Check sheet for the modelled part. Datum: model origin and axes. Units: mm. A direction names the side the tool comes from. Round coordinates to 2 decimals unless told otherwise and drop trailing zeros. Order: outer loops, then holes, each group sorted by start corner. A loop starts at its lowest first (then second) coordinate and runs counter-clockwise, first axis right, second up. Notation, with made-up numbers: (68.5, -28) -> (117.5, -28) arc R17 ccw to (117.5, -20) -> close; hole circle Ø1 at (-39.75, 12). An arc over 180 degrees is marked (long way). Answer in a Markdown table with one row per item.
```python
from build123d import *

# Parameters (mm, degrees)
SKETCH1_R           = 3.75
BOSS_EXTRUDE1_DEPTH = 8
SKETCH3_R           = 3.75
SKETCH3_R_2         = 3.25
CUT_EXTRUDE1_DEPTH  = 2
SKETCH4_R           = 1.75
CUT_EXTRUDE2_DEPTH  = 7.5
SKETCH5_R           = 2.5
CUT_EXTRUDE3_DEPTH  = 1


with BuildPart() as part:
    # Sketch1 → Boss-Extrude1 (new body)
    with BuildSketch(Plane(origin=(0, 0, 0), x_dir=(1, 0, 0), z_dir=(0, 1, 0))):
        Circle(SKETCH1_R)
    extrude(amount=BOSS_EXTRUDE1_DEPTH)

    # Sketch3 → Cut-Extrude1 (cut)
    with BuildSketch(Plane(origin=(0, 8, 0), x_dir=(1, 0, 0), z_dir=(0, 1, 0))):
        Circle(SKETCH3_R)
        Circle(SKETCH3_R_2, mode=Mode.SUBTRACT)
    extrude(amount=-CUT_EXTRUDE1_DEPTH, mode=Mode.SUBTRACT)

    # Sketch4 → Cut-Extrude2 (cut)
    with BuildSketch(Plane(origin=(0, 8, 0), x_dir=(1, 0, 0), z_dir=(0, 1, 0))):
        Circle(SKETCH4_R)
    extrude(amount=-CUT_EXTRUDE2_DEPTH, mode=Mode.SUBTRACT)

    # Sketch5 → Cut-Extrude3 (cut)
    with BuildSketch(Plane(origin=(0, 8, 0), x_dir=(1, 0, 0), z_dir=(0, 1, 0))):
        Circle(SKETCH5_R)
    extrude(amount=-CUT_EXTRUDE3_DEPTH, mode=Mode.SUBTRACT)


solid = part.part
```
(1) Section check B-B on y = 2. Record the boundary of the cut face in (x, z), plus the area to 3 significant figures.
Solutions:
| item | result |
|---|---|
| outline | circle Ø7.5 at (0, 0); hole circle Ø3.5 at (0, 0) |
| area | 34.6 mm^2 |
(2) Section check D-D on z = 2.75. Record the boundary of the cut face in (x, y).
Solutions:
| item | result |
|---|---|
| outline | (-2.55, 0) -> (2.55, 0) -> (2.55, 6) -> (1.73, 6) -> (1.73, 8) -> (-1.73, 8) -> (-1.73, 6) -> (-2.55, 6) -> close |
(3) Section check A-A on x = 0. Record the boundary of the cut face in (y, z).
Solutions:
| item | result |
|---|---|
| outline | (0, -3.75) -> (6, -3.75) -> (6, -3.25) -> (8, -3.25) -> (8, -2.5) -> (7, -2.5) -> (7, -1.75) -> (0.5, -1.75) -> (0.5, 1.75) -> (7, 1.75) -> (7, 2.5) -> (8, 2.5) -> (8, 3.25) -> (6, 3.25) -> (6, 3.75) -> (0, 3.75) -> close |
(4) Scan lines: probe 1 along Z at (x, y) = (0, 7.7); probe 2 along X at (y, z) = (1.25, 0). Record each from-to range of solid material in increasing order. Write a range as from..to.
Solutions:
| item | result |
|---|---|
| probe 1 | -3.25..-2.5, 2.5..3.25 |
| probe 2 | -3.75..-1.75, 1.75..3.75 |
(5) Draft check along Z on faces 1 (the flat face through (-1.4, 6, -3.1)), 2 (the cylindrical face through (-2.579, 7.014, 1.978)), 3 (the cylindrical face through (1.617, 3.796, 0.67)). Enter one of: pulls with the +Z half, pulls with the -Z half, needs draft (parallel to the pull), parting line crosses it, or undercut.
Solutions:
| item | result |
|---|---|
| face 1 | needs draft |
| face 2 | parting line crosses it |
| face 3 | undercut |
(6) Section check C-C on z = 0. Record the boundary of the cut face in (x, y), plus the area to 4 significant figures.
Solutions:
| item | result |
|---|---|
| outline | (-3.75, 0) -> (3.75, 0) -> (3.75, 6) -> (3.25, 6) -> (3.25, 8) -> (2.5, 8) -> (2.5, 7) -> (1.75, 7) -> (1.75, 0.5) -> (-1.75, 0.5) -> (-1.75, 7) -> (-2.5, 7) -> (-2.5, 8) -> (-3.25, 8) -> (-3.25, 6) -> (-3.75, 6) -> close |
| area | 30.25 mm^2 |
(7) Tool access check on faces 4 (the cylindrical face through (-0.54, 7.51, 2.44)), 5 (the flat face through (2, 8, 2)). Record the directions out of +Z, -Z, +X, -X, +Y, -Y that give a thin tool (end or side, any length) a straight path to the whole face; none if there is none.
Solutions:
| item | result |
|---|---|
| face 4 | +Y |
| face 5 | +Z, -Z, +X, -X, +Y |
(8) Depth check by flat-ended pin: pin 1 Ø3 at (x, y) = (3, 5) entering from -Z; pin 2 Ø4 at (x, y) = (2.5, 4.5) entering from -Z; pin 3 Ø4 at (x, z) = (0, 0) entering from -Y; pin 4 Ø1.8 at (x, z) = (0.5, 0.5) entering from +Y. Enter the tip coordinate at first touch or a pass-through.
Solutions:
| item | result |
|---|---|
| pin 1 | z = -3.44 |
| pin 2 | z = -3.72 |
| pin 3 | y = 0 |
| pin 4 | y = 0.5 |
